Part model, mm, in its own coordinate system. A direction names the side the tool comes from. Round coordinates to 2 decimals unless told otherwise and drop trailing zeros. Write each loop counter-clockwise with the first axis right and the second up, starting at its lowest first coordinate (ties: lowest second). Pieces come first, ordered by that corner, then holes.
1) Flat gauge pins, fed straight in: pin 1 (2 mm diameter, centred on x = 9.5, y = -5, fed in from +Z); pin 2 (3 mm diameter, centred on x = 18.5, z = -6.5, fed in from +Y); pin 3 (2 mm diameter, centred on y = -4, z = -4.5, fed in from +X); pin 4 (2 mm diameter, centred on x = 8, z = 0, fed in from +Y). Where does each tip first touch, or does it go through?
2) Saw through at C-C on z = 3. Write the cut outline in (x, y) (3 decimals).
3) Saw through at B-B on x = 66. Write the cut outline in (y, z) (3 decimals), and give its area (3 significant figures).
4) Pull direction Y, two halves, no side cores. Call faces 1 (the flat face through (8, -3, -8)), 2 (the flat face through (0, -2, 0)), 3 (the flat face through (69, -4.5, 6.3)): +Y half, -Y half, draft (parallel to the pull), parting line (faces both ways), or undercut.
5) Saw through at A-A on z = 0. Write the cut outline in (x, y) (3 decimals), and give its area (3 significant figures).
6) Drill centre lines: L1, parallel to X at y = -5.8, z = 3 (3 decimals); L2, parallel to X at y = -5.3, z = -8.5; L3, parallel to Z at x = 8, y = -1.8. Where is each one in solid material? Low to high.
7) Which spindle directions (+Z, -Z, +X, -X, +Y, -Y) get a long thin tool onto all of the face, cutting with end or side? Do faces 4 (the cylindrical face through (1.1, -2.6, 0.1)), 5 (the flat face through (69, -4.5, -6.3)), 6 (the flat face through (70, -3.925, 8)), 7 (the flat face through (8, -5, 7)). Say none if no direction does.
```python
from build123d import *

# Parameters (mm, degrees)
SKETCH1_W            = 20
SKETCH1_H            = 6
BOSS_EXTRUDE1_DEPTH  = 75
M3_CLEARANCE_HOLE1_D = 3.4
SKETCH4_R            = 1.975
CUT_EXTRUDE1_DEPTH   = 76.901251637
CUT_EXTRUDE2_DEPTH   = 10
SKETCH6_W            = 10
SKETCH6_H            = 3
CUT_EXTRUDE3_DEPTH   = 3
FILLET1_R            = 0.2
FILLET2_R            = 2.2
CUT_EXTRUDE5_DEPTH   = 2.2


with BuildPart() as part:
    # Sketch1 → Boss-Extrude1 (new body)
    with BuildSketch(Plane(origin=(0, 0, 0), x_dir=(0, 0, -1), z_dir=(1, 0, 0))):
        with Locations((0, -3)):
            Rectangle(SKETCH1_W, SKETCH1_H)
    extrude(amount=BOSS_EXTRUDE1_DEPTH)

    # M3 Clearance Hole1 (through all)
    with Locations(Plane(origin=(0, 0, 0), x_dir=(1, 0, 0), z_dir=(0, 1, 0))):
        with Locations((8, 0)):
            Hole(M3_CLEARANCE_HOLE1_D / 2)

    # Sketch4 → Cut-Extrude1 (cut, through all)
    with BuildSketch(Plane(origin=(0, 0, 0), x_dir=(1, 0, 0), z_dir=(0, 1, 0))):
        with Locations(Location((69.5, 3, 0), (0, 0, 270))):
            Circle(SKETCH4_R)
        with Locations(Location((69.5, -3, 0), (0, 0, 270))):
            Circle(SKETCH4_R)
    extrude(amount=-CUT_EXTRUDE1_DEPTH, mode=Mode.SUBTRACT)

    # Sketch5 → Cut-Extrude2 (cut)
    with BuildSketch(Plane(origin=(75, 0, 0), x_dir=(0, 0, -1), z_dir=(1, 0, 0))):
        Polygon((-10, -3.925), (-6.3, -3.925), (-6.3, -5.125), (6.3, -5.125), (6.3, -3.925), (10, -3.925), (10, -2.075), (6.3, -2.075), (6.3, -0.875), (-6.3, -0.875), (-6.3, -2.075), (-10, -2.075), align=None)
    extrude(amount=-CUT_EXTRUDE2_DEPTH, mode=Mode.SUBTRACT)

    # Sketch6 → Cut-Extrude3 (cut)
    with BuildSketch(Plane.XZ.offset(6)):
        with Locations((8, 8.5)):
            Rectangle(SKETCH6_W, SKETCH6_H)
        with Locations((8, -8.5)):
            Rectangle(SKETCH6_W, SKETCH6_H)
    extrude(amount=-CUT_EXTRUDE3_DEPTH, mode=Mode.SUBTRACT)

    # Fillet1
    fillet1_edges = [part.edges().sort_by_distance(p)[0] for p in [
        (3, -3, 8.5),
        (3, -4.5, 7),
        (8, -3, 10),
        (3, -4.5, 10),
        (13, -3, 8.5),
        (13, -4.5, 10),
        (8, -3, 7),
        (13, -4.5, 7),
        (3, -6, 8.5),
        (8, -6, 7),
        (13, -6, 8.5),
        (13, -3, -8.5),
        (13, -4.5, -7),
        (8, -3, -10),
        (13, -4.5, -10),
        (3, -3, -8.5),
        (3, -4.5, -10),
        (8, -3, -7),
        (3, -4.5, -7),
        (13, -6, -8.5),
        (8, -6, -7),
        (3, -6, -8.5),
    ]]
    fillet(fillet1_edges, radius=FILLET1_R)

    # Fillet2
    fillet2_edges = [part.edges().sort_by_distance(p)[0] for p in [
        (75, -1.475, -6.3),
        (75, -1.475, 6.3),
        (75, -4.525, 6.3),
        (75, -4.525, -6.3),
    ]]
    fillet(fillet2_edges, radius=FILLET2_R)

    # Sketch12 → Cut-Extrude5 (cut)
    with BuildSketch(Plane.ZY):
        with BuildLine():
            ThreePointArc((10, -5.554612339), (0, -2.6), (-10, -5.554612339))
            Line((-10, -5.554612339), (-10, -6))
            Line((-10, -6), (10, -6))
            Line((10, -6), (10, -5.554612339))
        make_face()
        with BuildLine():
            Line((-10, -6), (-10, -5.554612339))
            ThreePointArc((-10, -5.554612339), (-8.79090439, -37.164157881), (18.4, -21))
            ThreePointArc((18.4, -21), (16.164157881, -12.20909561), (10, -5.554612339))
            Line((10, -5.554612339), (10, -6))
            Line((10, -6), (-10, -6))
        make_face()
    extrude(amount=-CUT_EXTRUDE5_DEPTH, mode=Mode.SUBTRACT)


solid = part.part
```
Completed:
1. pin 1: stops at z = 7
1. pin 2: stops at y = 0
1. pin 3: stops at x = 65
1. pin 4: passes through
2. outline: (0, -2.846) - (2.2, -2.846) - (2.2, -6) - (67.525, -6) - (67.525, -5.125) - (65, -5.125) - (65, -0.875) - (67.525, -0.875) - (67.525, 0) - (0, 0) - close; (71.475, -6) - (75, -6) - (75, -5.125) - (71.475, -5.125) - close; (71.475, -0.875) - (75, -0.875) - (75, 0) - (71.475, 0) - close
3. outline: (-6, -10) - (-3.925, -10) - (-3.925, -6.3) - (-5.125, -6.3) - (-5.125, 6.3) - (-3.925, 6.3) - (-3.925, 10) - (-6, 10) - close; (-2.075, -10) - (0, -10) - (0, 10) - (-2.075, 10) - (-2.075, 6.3) - (-0.875, 6.3) - (-0.875, -6.3) - (-2.075, -6.3) - close
3. area: 52.8 mm2
4. face 1: -Y half
4. face 2: draft
4. face 3: undercut
5. outline: (0, -2.6) - (2.2, -2.6) - (2.2, -6) - (6.3, -6) - (6.3, 0) - (0, 0) - close; (9.7, -6) - (75, -6) - (75, -5.125) - (65, -5.125) - (65, -0.875) - (75, -0.875) - (75, 0) - (9.7, 0) - close
5. area: 380 mm2
6. L1: x = 2.2 to 67.525, 71.475 to 75
6. L2: x = 2.2 to 3, 13 to 75
6. L3: z = -10 to -1.7, 1.7 to 10
7. face 4: -X, -Y
7. face 5: +X
7. face 6: +Z, -Z, +X
7. face 7: +Z, -Y
